Check sheet for the modelled part. Datum: model origin and axes. Units: mm. A direction names the side the tool comes from. Round coordinates to 2 decimals unless told otherwise and drop trailing zeros. Loops run counter-clockwise (first coordinate to the right, second up) from the corner with the lowest first, then second, coordinate; pieces in that order, holes last. Notation, with made-up numbers: (-34, 26) - (-1, 26) arc R34 cw to (-1, 64) - close; hole circle Ø7 at (-8.5, 46.25). An arc over 180 degrees is marked (long way). Answer in a Markdown table with one row per item. Add a question column.
(1) Access from +Z, -Z, +X, -X, +Y, -Y to the whole of each face (thin tool, end or side, straight path). Record for faces 4 (the cylindrical face through (39.47, 16.07, -44.19)), 5 (the flat face through (-1, 3.175, 1)), 6 (the flat face through (-5, 2, 39.684)).
(2) Thickness scan on line 1 along X through (y, z) = (17, -28) (3 decimals); line 2 along Y through (x, z) = (0, -44.15); line 3 along X through (y, z) = (2.85, 38.1) (3 decimals). Record the ranges inside material, lowest first.
(3) Cross-section at C-C on x = -24. Enter the section's corners in (y, z) (3 decimals).
(4) Gauge pin test, flat ends, axial feed: pin 1 (10 mm diameter, centred on x = -25, z = 27.5, fed in from +Y) (3 decimals); pin 2 (6 mm diameter, centred on x = -31, y = 15, fed in from +Z) (3 decimals). Record the tip position at first contact, or that the pin passes through.
(5) Cross-section at B-B on z = 6.5. Enter the section's corners in (x, y) (3 decimals), then the cut area to 3 significant figures.
(6) Cross-section at D-D on z = -13. Enter the section's corners in (x, y) (3 decimals).
(7) Mould release check, pull along Z, two halves, no side actions. Record for faces 1 (the conical face through (28.37, 1.77, 39.58)), 2 (the flat face through (-57.15, 9, -12)), 3 (the conical face through (2.1, 13.2, -43.8)): +Z half, -Z half, draft (parallel to the pull), parting line (faces both ways), or undercut.
(8) Cross-section at A-A on x = 46.93. Count the separate pieces of the cut face and the enclosed holes in it, then the cut area to 3 significant figures.
from build123d import *

# Parameters (mm, degrees)
SKETCH1_W                                     = 120.65
SKETCH1_H                                     = 88.9
BOSS_EXTRUDE1_DEPTH                           = 3.175
SKETCH2_W                                     = 120.65
SKETCH2_H                                     = 3.175
BOSS_EXTRUDE2_DEPTH                           = 22.225
CSK_FOR_6_FLAT_HEAD_MACHINE_SCREW1_AT_2_COUNT = 2
CSK_FOR_6_FLAT_HEAD_MACHINE_SCREW1_AT_2_PITCH = 71
CSK_FOR_6_FLAT_HEAD_MACHINE_SCREW1_AT_3_COUNT = 2
CSK_FOR_6_FLAT_HEAD_MACHINE_SCREW1_AT_3_PITCH = 100.409162928
CSK_FOR_6_FLAT_HEAD_MACHINE_SCREW1_AT_4_COUNT = 2
CSK_FOR_6_FLAT_HEAD_MACHINE_SCREW1_AT_4_PITCH = 71
CUT_EXTRUDE1_DEPTH                            = 80.120592294
FILLET2_R                                     = 3.175
BOSS_EXTRUDE3_DEPTH                           = 3.175
FILLET3_R                                     = 6.35
FILLET3_OF_MIRROR1_R                          = 6.35
CSK_FOR_8_FLAT_HEAD_SOCKET_CAP_SCREW1_A_COUNT = 2
CSK_FOR_8_FLAT_HEAD_SOCKET_CAP_SCREW1_A_PITCH = 76.2
CSK_FOR_8_FLAT_HEAD_SOCKET_CAP_SCRE_2_COUNT   = 2
CSK_FOR_8_FLAT_HEAD_SOCKET_CAP_SCRE_2_PITCH   = 38.1
CUT_EXTRUDE2_REACH                            = 80.159
SKETCH12_R                                    = 7.9375


with BuildPart() as part:
    # Sketch1 → Boss-Extrude1 (new body)
    with BuildSketch(Plane(origin=(0, 0, 0), x_dir=(1, 0, 0), z_dir=(0, 1, 0))):
        Rectangle(SKETCH1_W, SKETCH1_H)
    extrude(amount=BOSS_EXTRUDE1_DEPTH)

    # Sketch2 → Boss-Extrude2 (add)
    with BuildSketch(Plane(origin=(0, 3.175, 0), x_dir=(1, 0, 0), z_dir=(0, 1, 0))):
        with Locations((0, 42.8625)):
            Rectangle(SKETCH2_W, SKETCH2_H)
    extrude(amount=BOSS_EXTRUDE2_DEPTH)

    # Sketch4 → CSK for #6 Flat Head Machine Screw1 (revolve, cut)
    with BuildSketch(Plane(origin=(29.725, 0, 38.1), x_dir=(0, 0, -1), z_dir=(1, 0, 0))):
        Polygon((0, 0), (0, 3.175), (1.89865, 3.175), (1.89865, 1.891953401), (3.5433, 0), align=None)
    csk_for_6_flat_head_machine_screw1 = revolve(axis=Axis((29.725, -6.35, 38.1), (0, 1, 0)), mode=Mode.SUBTRACT)

    # CSK for #6 Flat Head Machine Screw1 at 2: CSK for #6 Flat Head Machine Screw1 ×2
    with Locations(*[(0, 0, -i * CSK_FOR_6_FLAT_HEAD_MACHINE_SCREW1_AT_2_PITCH) for i in range(1, CSK_FOR_6_FLAT_HEAD_MACHINE_SCREW1_AT_2_COUNT)]):
        add(csk_for_6_flat_head_machine_screw1, mode=Mode.SUBTRACT)

    # CSK for #6 Flat Head Machine Screw1 at 3: CSK for #6 Flat Head Machine Screw1 ×2
    with Locations(*[Vector(-0.7071067811865476, 0, -0.7071067811865476) * (i * CSK_FOR_6_FLAT_HEAD_MACHINE_SCREW1_AT_3_PITCH) for i in range(1, CSK_FOR_6_FLAT_HEAD_MACHINE_SCREW1_AT_3_COUNT)]):
        add(csk_for_6_flat_head_machine_screw1, mode=Mode.SUBTRACT)

    # CSK for #6 Flat Head Machine Screw1 at 4: CSK for #6 Flat Head Machine Screw1 ×2
    with Locations(*[(-i * CSK_FOR_6_FLAT_HEAD_MACHINE_SCREW1_AT_4_PITCH, 0, 0) for i in range(1, CSK_FOR_6_FLAT_HEAD_MACHINE_SCREW1_AT_4_COUNT)]):
        add(csk_for_6_flat_head_machine_screw1, mode=Mode.SUBTRACT)

    # Sketch6 → Cut-Extrude1 (cut, through all)
    with BuildSketch(Plane.XZ):
        Polygon((-47.05, -21.784), (-42.608645627, -26.225354373), (-10.525631341, 2.6), (-42.608645627, 31.425354373), (-47.05, 26.984), align=None)
        Polygon((-38.112099916, 35.921900084), (-5.775, 6.868259544), (26.562099916, 35.921900084), (22.8, 39.684), (-34.35, 39.684), align=None)
        Polygon((-1.024368659, 2.6), (31.058645627, -26.225354373), (35.5, -21.784), (35.5, 26.984), (31.058645627, 31.425354373), align=None)
        Polygon((-38.112099916, -30.721900084), (-5.775, -1.668259544), (26.562099916, -30.721900084), (22.8, -34.484), (-34.35, -34.484), align=None)
    extrude(amount=-CUT_EXTRUDE1_DEPTH, mode=Mode.SUBTRACT)

    # Fillet2
    fillet2_edges = [part.edges().sort_by_distance(p)[0] for p in [
        (31.058645627, 1.5875, -26.225354373),
        (-1.024368659, 1.5875, 2.6),
        (31.058645627, 1.5875, 31.425354373),
        (35.5, 1.5875, 26.984),
        (35.5, 1.5875, -21.784),
        (-38.112099916, 1.5875, -30.721900084),
        (-5.775, 1.5875, -1.668259544),
        (26.562099916, 1.5875, -30.721900084),
        (22.8, 1.5875, -34.484),
        (-34.35, 1.5875, -34.484),
        (-42.608645627, 1.5875, -26.225354373),
        (-47.05, 1.5875, -21.784),
        (-47.05, 1.5875, 26.984),
        (-42.608645627, 1.5875, 31.425354373),
        (-10.525631341, 1.5875, 2.6),
        (-5.775, 1.5875, 6.868259544),
        (-38.112099916, 1.5875, 35.921900084),
        (-34.35, 1.5875, 39.684),
        (22.8, 1.5875, 39.684),
        (26.562099916, 1.5875, 35.921900084),
    ]]
    fillet(fillet2_edges, radius=FILLET2_R)

    # Sketch9 → Boss-Extrude3 (add)
    with BuildSketch(Plane.ZY.offset(60.325)):
        Polygon((-41.275, 25.4), (44.45, 3.175), (-41.275, 3.175), align=None)
    boss_extrude3 = extrude(amount=-BOSS_EXTRUDE3_DEPTH)

    # Fillet3
    fillet3_edges = [part.edges().sort_by_distance(p)[0] for p in [
        (-57.15, 14.2875, -41.275),
    ]]
    fillet(fillet3_edges, radius=FILLET3_R)

    # Mirror1: Boss-Extrude3 across plane
    add(boss_extrude3.mirror(Plane(origin=(0, 0, 0), x_dir=(0, 0, 1), z_dir=(1, 0, 0))))

    # Fillet3 of Mirror1
    fillet3_of_mirror1_edges = [part.edges().sort_by_distance(p)[0] for p in [
        (57.15, 14.2875, -41.275),
    ]]
    fillet(fillet3_of_mirror1_edges, radius=FILLET3_OF_MIRROR1_R)

    # Sketch10 → CSK for #8 Flat Head Socket Cap Screw1 (revolve, cut)
    with BuildSketch(Plane(origin=(-38.1, 14.2875, -41.275), x_dir=(0, -1, 0), z_dir=(1, 0, 0))):
        Polygon((0, 0), (0, 3.175), (2.2479, 3.175), (2.2479, 2.658961536), (4.5593, 0), align=None)
    csk_for_8_flat_head_socket_cap_screw1 = revolve(axis=Axis((-38.1, 14.2875, -34.925), (0, 0, -1)), mode=Mode.SUBTRACT)

    # CSK for #8 Flat Head Socket Cap Screw1 a: CSK for #8 Flat Head Socket Cap Screw1 ×2
    with Locations(*[(i * CSK_FOR_8_FLAT_HEAD_SOCKET_CAP_SCREW1_A_PITCH, 0, 0) for i in range(1, CSK_FOR_8_FLAT_HEAD_SOCKET_CAP_SCREW1_A_COUNT)]):
        add(csk_for_8_flat_head_socket_cap_screw1, mode=Mode.SUBTRACT)

    # CSK for _8 Flat Head Socket Cap Scre 2: CSK for #8 Flat Head Socket Cap Screw1 ×2
    with Locations(*[(i * CSK_FOR_8_FLAT_HEAD_SOCKET_CAP_SCRE_2_PITCH, 0, 0) for i in range(1, CSK_FOR_8_FLAT_HEAD_SOCKET_CAP_SCRE_2_COUNT)]):
        add(csk_for_8_flat_head_socket_cap_screw1, mode=Mode.SUBTRACT)

    # Sketch12 → Cut-Extrude2 (cut, up to next)
    with BuildSketch(Plane(origin=(0, 3.175, 0), x_dir=(1, 0, 0), z_dir=(0, 1, 0)), mode=Mode.PRIVATE) as cut_extrude2_sk1:
        with Locations(Location((46.93, 27.88, 0), (0, 0, 270))):
            Circle(SKETCH12_R)
    cut_extrude2_tool1 = extrude(cut_extrude2_sk1.sketch, amount=-CUT_EXTRUDE2_REACH, mode=Mode.PRIVATE) & part.part
    # Sketch12 → Cut-Extrude2 (cut, up to next)
    with BuildSketch(Plane(origin=(0, 3.175, 0), x_dir=(1, 0, 0), z_dir=(0, 1, 0)), mode=Mode.PRIVATE) as cut_extrude2_sk2:
        with Locations(Location((46.93, 7.56, 0), (0, 0, 270))):
            Circle(SKETCH12_R)
    cut_extrude2_tool2 = extrude(cut_extrude2_sk2.sketch, amount=-CUT_EXTRUDE2_REACH, mode=Mode.PRIVATE) & part.part
    # Sketch12 → Cut-Extrude2 (cut, up to next)
    with BuildSketch(Plane(origin=(0, 3.175, 0), x_dir=(1, 0, 0), z_dir=(0, 1, 0)), mode=Mode.PRIVATE) as cut_extrude2_sk3:
        with Locations(Location((46.93, -12.76, 0), (0, 0, 270))):
            Circle(SKETCH12_R)
    cut_extrude2_tool3 = extrude(cut_extrude2_sk3.sketch, amount=-CUT_EXTRUDE2_REACH, mode=Mode.PRIVATE) & part.part
    # Sketch12 → Cut-Extrude2 (cut, up to next)
    with BuildSketch(Plane(origin=(0, 3.175, 0), x_dir=(1, 0, 0), z_dir=(0, 1, 0)), mode=Mode.PRIVATE) as cut_extrude2_sk4:
        with Locations(Location((46.93, -33.08, 0), (0, 0, 270))):
            Circle(SKETCH12_R)
    cut_extrude2_tool4 = extrude(cut_extrude2_sk4.sketch, amount=-CUT_EXTRUDE2_REACH, mode=Mode.PRIVATE) & part.part
    add(cut_extrude2_tool1.solids().sort_by_distance((46.93, 3.175, -27.88))[0], mode=Mode.SUBTRACT)
    add(cut_extrude2_tool2.solids().sort_by_distance((46.93, 3.175, -7.56))[0], mode=Mode.SUBTRACT)
    add(cut_extrude2_tool3.solids().sort_by_distance((46.93, 3.175, 12.76))[0], mode=Mode.SUBTRACT)
    add(cut_extrude2_tool4.solids().sort_by_distance((46.93, 3.175, 33.08))[0], mode=Mode.SUBTRACT)


solid = part.part
Answers:
| question | item | result |
|---|---|---|
| 1 | face 4 | +Z, -Z |
| 1 | face 5 | +Z, +Y |
| 1 | face 6 | +Y, -Y |
| 2 | line 1 | x = -60.325 to -57.15, 57.15 to 60.325 |
| 2 | line 2 | y = 0 to 12.04, 16.54 to 25.4 |
| 2 | line 3 | x = -60.325 to -43.174, -39.376 to -35.919, 24.369 to 27.826, 31.624 to 40.782, 53.078 to 60.325 |
| 3 | outline | (0, -44.45) - (25.4, -44.45) - (25.4, -41.275) - (3.175, -41.275) - (3.175, -34.484) - (0, -34.484) - close; (0, -18.043) - (3.175, -18.043) - (3.175, -9.506) - (0, -9.506) - close; (0, 14.706) - (3.175, 14.706) - (3.175, 23.243) - (0, 23.243) - close; (0, 39.684) - (3.175, 39.684) - (3.175, 44.45) - (0, 44.45) - close |
| 4 | pin 1 | stops at y = 3.175 |
| 4 | pin 2 | stops at z = -41.275 |
| 5 | outline | (-60.325, 0) - (-47.05, 0) - (-47.05, 3.175) - (-57.15, 3.175) - (-57.15, 13.014) - (-60.325, 13.014) - close; (-14.866, 0) - (3.316, 0) - (3.316, 3.175) - (-14.866, 3.175) - close; (35.5, 0) - (42.05, 0) - (42.05, 3.175) - (35.5, 3.175) - close; (51.81, 0) - (60.325, 0) - (60.325, 13.014) - (57.15, 13.014) - (57.15, 3.175) - (51.81, 3.175) - close |
| 5 | area | 210 mm^2 |
| 6 | outline | (-60.325, 0) - (-47.05, 0) - (-47.05, 3.175) - (-57.15, 3.175) - (-57.15, 18.069) - (-60.325, 18.069) - close; (-27.889, 0) - (-18.387, 0) - (-18.387, 3.175) - (-27.889, 3.175) - close; (6.837, 0) - (16.339, 0) - (16.339, 3.175) - (6.837, 3.175) - close; (35.5, 0) - (41.15, 0) - (41.15, 3.175) - (35.5, 3.175) - close; (52.71, 0) - (60.325, 0) - (60.325, 18.069) - (57.15, 18.069) - (57.15, 3.175) - (52.71, 3.175) - close |
| 7 | face 1 | undercut |
| 7 | face 2 | draft |
| 7 | face 3 | +Z half |
| 8 | separate pieces | 5 |
| 8 | enclosed holes | 0 |
| 8 | area | 151 mm^2 |
